Work out the finished part from the listing and answer in its coordinate system (mm). A direction names the side the tool comes from. Coordinates: 2 decimals unless noted, no trailing zeros. Order: outer loops, then holes, each group sorted by start corner. A loop starts at its lowest first (then second) coordinate and runs counter-clockwise, first axis right, second up. Notation, with made-up numbers: M -8,37.5 L 18,37.5 A30 ccw 18,75.5 Z; hole C -4.5,77 d11. An arc over 180 degrees is marked long. Use a Markdown table: item, result.
Autodesk Inventor part; units mm, degrees
ref_plane "YZ Plane" through (0, 0, 0) normal (1, 0, 0) x (0, 1, 0)
ref_plane "XZ Plane" through (0, 0, 0) normal (0, 1, 0) x (-1, 0, 0)
ref_plane "XY Plane" through (0, 0, 0) normal (0, 0, 1) x (1, 0, 0)
sketch "Sketch1" plane through (0, 0, 0) normal (0, 0, 1) x (1, 0, 0)
  circle A0 centre (0, 0) radius 5
  circle A1 centre (0, 0) radius 2.5
  dimension "d0" = 10
  dimension "d1" = 5
extrude "Extrusion1" add sketch "Sketch1" along normal blind 25
sketch "Sketch2" plane through (0, 0, 25) normal (0, 0, 1) x (1, 0, 0)
  line L0 (0, 20) -> (38, 20)
  line L1 (38, 20) -> (38, -20)
  line L2 (38, -20) -> (-38, -20)
  line L3 (-38, -20) -> (-38, 20)
  line L4 (-38, 20) -> (0, 20)
  circle A0 centre (0, 0) radius 2.5
  dimension "d4" = 20
  dimension "d6" = 38
  dimension "d7" = 40
  dimension "d8" = 76
  dimension "d9" = 40
extrude "Extrusion2" add sketch "Sketch2" along normal blind 10
sketch "Sketch3" plane through (0, 0, 35) normal (0, 0, 1) x (1, 0, 0)
  line L0 (38, 20) -> (-38, 20)
  line L1 (38, 20) -> (43, 20)
  line L2 (43, 20) -> (43, -20)
  line L3 (43, -20) -> (38, -20)
  line L4 (38, -20) -> (38, 20)
  line L5 (-38, 20) -> (-38, -20)
  line L6 (-38, -20) -> (-43, -20)
  line L7 (-43, -20) -> (-43, 20)
  line L8 (-43, 20) -> (-38, 20)
  line L9 (-38, 20) -> (-38, -20)
  point P0 (0, 0)
  dimension "d12" = 5
  dimension "d13" = 40
  dimension "d14" = 5
extrude "Extrusion3" add sketch "Sketch3" along normal blind 15 and the other way blind 10
sketch "Sketch4" plane through (-38, -20, 35) normal (1, 0, 0) x (0, 0, -1)
  point P0 (35, 20)
sketch "Sketch5" plane through (-38, -20, 35) normal (1, 0, 0) x (0, 0, -1)
  line L0 (0, 0) -> (-15, 0)
  line L1 (-14.9948, 39.7098) -> (-11.9948, 39.7098)
  line L2 (-11.9948, 39.7098) -> (-11.9948, 0)
  line L3 (-11.9948, 0) -> (-14.9948, 0)
  line L4 (-14.9948, 0) -> (-14.9948, 39.7098)
  point P0 (35, 20)
  dimension "d19" = 3
extrude "Extrusion4" add sketch "Sketch5" along normal blind 5
sketch "Sketch6" plane through (38, -20, 35) normal (-1, 0, 0) x (0, 0, 1)
  line L0 (11.9948, 39.7098) -> (14.9948, 39.7098)
  line L1 (11.9948, 39.7098) -> (11.9948, 0)
  line L2 (14.9948, 39.7098) -> (11.9948, 39.7098)
  line L3 (11.9948, 39.7098) -> (11.9948, 0)
  line L4 (11.9948, 0) -> (14.9948, 0)
  line L5 (14.9948, 0) -> (14.9948, 39.7098)
  point P0 (-35, 20)
extrude "Extrusion5" add sketch "Sketch6" along normal blind 5
sketch "Sketch11" plane through (-43, 20, 25) normal (0, 1, 0) x (1, 0, 0)
  line L0 (5, -10) -> (81, -10)
  line L1 (86, 0) -> (0, 0)
  line L2 (56, -10) -> (71, -10)
  line L3 (71, -10) -> (71, 0)
  line L4 (71, 0) -> (56, 0)
  line L5 (56, 0) -> (56, -10)
  point P0 (43, 25)
  dimension "d39" = 15
extrude "Extrusion8" add sketch "Sketch11" along normal blind 85
sketch "Sketch12" plane through (0, 0, 35) normal (0, 0, 1) x (1, 0, 0)
  line L0 (13, 20) -> (13, 105)
  line L1 (13, 105) -> (13, 100)
  line L2 (13, 100) -> (28, 100)
  line L3 (28, 100) -> (28, 105)
  line L4 (28, 105) -> (13, 105)
  point P0 (0, 0)
  dimension "d42" = 5
  dimension "d43" = 15
extrude "Extrusion9" add sketch "Sketch12" along normal blind 15
sketch "Sketch13" plane through (13, 100, 35) normal (0, -1, 0) x (1, 0, 0)
  line L0 (0, -10) -> (0, 15)
  line L1 (0, 15) -> (0, 12)
  line L2 (0, 12) -> (15, 12)
  line L3 (15, 12) -> (15, 15)
  line L4 (15, 15) -> (0, 15)
  point P0 (-13, -35)
  dimension "d46" = 3
  dimension "d47" = 15
extrude "Extrusion10" add sketch "Sketch13" along normal blind 5
sketch "Sketch14" plane through (-43, -20, 25) normal (0, -1, 0) x (1, 0, 0)
  line L0 (0, 0) -> (86, 0)
  line L1 (43, 0) -> (31, 0)
  point P0 (43, -25)
  point P1 (56, 0)
  dimension "d50" = 12
sketch "Sketch15" plane through (-43, -20, 25) normal (0, -1, 0) x (1, 0, 0)
  line L0 (48, 0) -> (38, 0)
  line L1 (43, 0) -> (31, 0)
  line L2 (31, 0) -> (31, 3)
  line L3 (31, 3) -> (16, 3)
  line L4 (16, 3) -> (16, 7)
  line L5 (16, 7) -> (31, 7)
  line L6 (31, 7) -> (31, 3)
  point P0 (43, -25)
  dimension "d51" = 12
  dimension "d52" = 3
  dimension "d53" = 15
  dimension "d54" = 4
extrude "Extrusion11" cut sketch "Sketch15" against normal blind 15
properties part number "Holder"
1. Flat-ended cylindrical pins translate along their axes: P1, Ø12, axis at x = -19, y = -9, coming from the -Z side; P2, Ø12.5, axis at y = 45.5, z = 37.5, coming from the -X side; P3, Ø1.5, axis at x = 22.5, z = 48, coming from the -Y side. Find the tip coordinate at first contact, or state that the pin passes through.
Answers below:
| item | result |
|---|---|
| P1 | z = 25 |
| P2 | x = 13 |
| P3 | y = 95 |
2. Section C-C on z = 40 is taken. Determine the outline of the cut face in (x, y), then the cut area to 3 significant figures.
Answers below:
| item | result |
|---|---|
| outline | M -43,-20 L -38,-20 L -38,20 L -43,20 Z; M 13,100 L 28,100 L 28,105 L 13,105 Z; M 38,-20 L 43,-20 L 43,20 L 38,20 Z |
| area | 475 mm² |
3. For faces 5 (the face through (20, 95, 49)), 6 (the face through (-15, 20, 32)), 7 (the face through (-36, 19.71, 49)), 8 (the face through (-20, -5, 30)), 9 (the face through (20, 100, 41)), determine the directions among +Z, -Z, +X, -X, +Y, -Y from which every point of the face is accessible in a straight line to the end or side of a thin tool.
Answers below:
| item | result |
|---|---|
| face 5 | +Z, +X, -X, -Y |
| face 6 | +Z, -Z, -X, +Y |
| face 7 | +Z, +Y |
| face 8 | -Y |
| face 9 | +X, -X, -Y |
4. Section A-A on x = 0 is taken. Determine the outline of the cut face in (y, z).
Answers below:
| item | result |
|---|---|
| outline | M -20,25 L -5,25 L -5,0 L -2.5,0 L -2.5,35 L -20,35 Z; M 2.5,0 L 5,0 L 5,25 L 20,25 L 20,35 L 2.5,35 Z |
5. Find the intervals of material crossed by probe 1 along X at (y, z) = (19.5, 44.5); probe 2 along Z at (x, y) = (-20.5, -11); probe 3 along Y at (x, z) = (0, 13), in increasing order.
Answers below:
| item | result |
|---|---|
| probe 1 | -43 to -38, 38 to 43 |
| probe 2 | 25 to 28, 32 to 35 |
| probe 3 | -5 to -2.5, 2.5 to 5 |
6. Section D-D on x = -25 is taken. Determine the outline of the cut face in (y, z).
Answers below:
| item | result |
|---|---|
| outline | M -20,25 L 20,25 L 20,35 L -20,35 L -20,32 L -5,32 L -5,28 L -20,28 Z |
7. For a pull along Z with two mould halves and no side action, classify faces 1 (the face through (-36, 0, 46.995)), 2 (the face through (21, 100, 50)), 3 (the face through (-12, -13, 30)), 4 (the face through (13, 63, 32)) as +Z half, -Z half, draft (parallel to the pull), parting line (faces both ways), or undercut.
Answers below:
| item | result |
|---|---|
| face 1 | undercut |
| face 2 | +Z half |
| face 3 | undercut |
| face 4 | draft |
